Geometry: final body of the model. Coordinates: model frame, mm. Give positions to 0.01 mm unless a question says otherwise; leave off trailing zeros. Order: outer loops, then holes, each group sorted by start corner. A loop starts at its lowest first (then second) coordinate and runs counter-clockwise, first axis right, second up. Notation, with made-up numbers: (-7, 13.25) -> (22, 13.25) arc R8 ccw to (22, 23.25) -> close; hole circle Ø11 at (79.5, -3). An arc over 180 degrees is marked (long way). Answer in a Markdown table with one row per item. Add a question column.
Q1. Cut plane C-C on x = -42. Return the cut outline in (y, z), and give its area (3 significant figures).
Q2. Line query: line 1 along X through (y, z) = (3.7, 52); line 2 along X through (y, z) = (2.5, 130.5); line 3 along Z through (x, y) = (-10.5, 1.55). Output: solid intervals per line, ascending. Write a range as from..to.
Q3. Cut plane A-A on z = 45. Return the cut outline in (x, y).
Q4. Cut plane B-B on x = 21.5. Return the cut outline in (y, z), and give its area (3 significant figures).
Q5. Contact query for flat-ended pins moving along their axis: P1, Ø1.5, axis at y = 2, z = 129, coming from the +X side; P2, Ø3, axis at x = -34.5, y = 1.5, coming from the +Z side; P3, Ø2.5, axis at x = 0.5, y = 3.5, coming from the -Z side. Output: stop coordinate, or through.
Q6. Cut plane D-D on z = 73. Return the cut outline in (x, y).
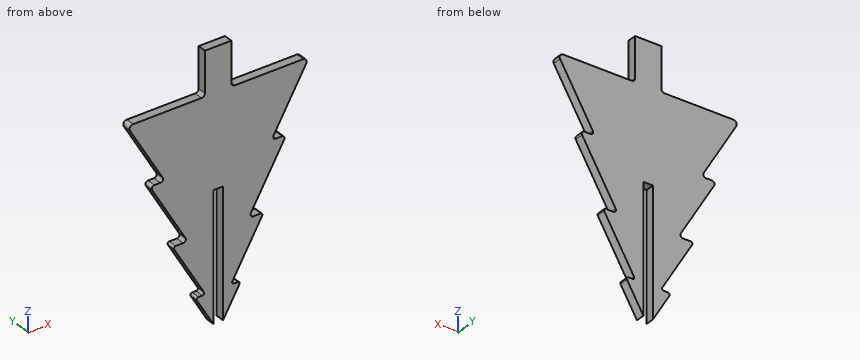
from build123d import *

# Parameters (mm, degrees)
ESBO_O1_W     = 15
ESBO_O1_H     = 25
RVORE_DEPTH   = 5
ESBO_O3_W     = 5.5
ESBO_O3_H     = 77.5
ENCAIXE_DEPTH = 5
FILETE1_R     = 1.5
FILETE2_R     = 1
FILETE3_R     = 1.5
FILETE4_R     = 1.5
FILETE5_R     = 2
FILETE6_R     = 1
FILETE7_R     = 1
FILETE8_R     = 2
FILETE9_R     = 1.5
FILETE10_R    = 1.5
FILETE11_R    = 1.5
FILETE12_R    = 1
FILETE13_R    = 1
FILETE14_R    = 1
FILETE15_R    = 2
FILETE16_R    = 2


with BuildPart() as part:
    # Esboço1 → rvore (new body)
    with BuildSketch(Plane(origin=(0, 0, 0), x_dir=(1, 0, 0), z_dir=(0, 1, 0))):
        with Locations((0, -127.5)):
            Rectangle(ESBO_O1_W, ESBO_O1_H)
        Polygon((-51.961524227, -115), (-7.5, -115), (7.5, -115), (51.961524227, -115), (30.310889132, -77.5), (-30.310889132, -77.5), align=None)
        Polygon((-8.660254038, -40), (-30.310889132, -77.5), (30.310889132, -77.5), (8.660254038, -40), align=None)
        Polygon((-17.320508076, -40), (-8.660254038, -40), (0, -25), (8.660254038, -40), (17.320508076, -40), (0, -10), align=None)
        Polygon((8.660254038, -40), (30.310889132, -77.5), (38.97114317, -77.5), (17.320508076, -40), align=None)
        Polygon((0, -25), (-8.660254038, -40), (8.660254038, -40), align=None)
        Polygon((-38.97114317, -77.5), (-30.310889132, -77.5), (-8.660254038, -40), (-17.320508076, -40), align=None)
        Polygon((-25.980762114, -40), (-17.320508076, -40), (0, -10), (17.320508076, -40), (25.980762114, -40), (7.216878365, -7.5), (-7.216878365, -7.5), align=None)
        Polygon((0, 5), (-7.216878365, -7.5), (7.216878365, -7.5), align=None)
        Polygon((-12.990381057, -7.5), (-7.216878365, -7.5), (0, 5), (7.216878365, -7.5), (12.990381057, -7.5), (0, 15), align=None)
    extrude(amount=RVORE_DEPTH)

    # Esboço3 → Encaixe (cut)
    with BuildSketch(Plane(origin=(0, 5, 0), x_dir=(1, 0, 0), z_dir=(0, 1, 0))):
        with Locations((0, -23.75)):
            Rectangle(ESBO_O3_W, ESBO_O3_H)
    extrude(amount=-ENCAIXE_DEPTH, mode=Mode.SUBTRACT)

    # Filete1
    filete1_edges = [part.edges().sort_by_distance(p)[0] for p in [
        (17.320508076, 2.5, 40),
    ]]
    fillet(filete1_edges, radius=FILETE1_R)

    # Filete2
    filete2_edges = [part.edges().sort_by_distance(p)[0] for p in [
        (25.980762114, 2.5, 40),
    ]]
    fillet(filete2_edges, radius=FILETE2_R)

    # Filete3
    filete3_edges = [part.edges().sort_by_distance(p)[0] for p in [
        (38.97114317, 2.5, 77.5),
    ]]
    fillet(filete3_edges, radius=FILETE3_R)

    # Filete4
    filete4_edges = [part.edges().sort_by_distance(p)[0] for p in [
        (30.310889132, 2.5, 77.5),
    ]]
    fillet(filete4_edges, radius=FILETE4_R)

    # Filete5
    filete5_edges = [part.edges().sort_by_distance(p)[0] for p in [
        (51.961524227, 2.5, 115),
    ]]
    fillet(filete5_edges, radius=FILETE5_R)

    # Filete6
    filete6_edges = [part.edges().sort_by_distance(p)[0] for p in [
        (12.990381057, 2.5, 7.5),
    ]]
    fillet(filete6_edges, radius=FILETE6_R)

    # Filete7
    filete7_edges = [part.edges().sort_by_distance(p)[0] for p in [
        (7.216878365, 2.5, 7.5),
    ]]
    fillet(filete7_edges, radius=FILETE7_R)

    # Filete8
    filete8_edges = [part.edges().sort_by_distance(p)[0] for p in [
        (-51.961524227, 2.5, 115),
    ]]
    fillet(filete8_edges, radius=FILETE8_R)

    # Filete9
    filete9_edges = [part.edges().sort_by_distance(p)[0] for p in [
        (-30.310889132, 2.5, 77.5),
    ]]
    fillet(filete9_edges, radius=FILETE9_R)

    # Filete10
    filete10_edges = [part.edges().sort_by_distance(p)[0] for p in [
        (-38.97114317, 2.5, 77.5),
    ]]
    fillet(filete10_edges, radius=FILETE10_R)

    # Filete11
    filete11_edges = [part.edges().sort_by_distance(p)[0] for p in [
        (-17.320508076, 2.5, 40),
    ]]
    fillet(filete11_edges, radius=FILETE11_R)

    # Filete12
    filete12_edges = [part.edges().sort_by_distance(p)[0] for p in [
        (-25.980762114, 2.5, 40),
    ]]
    fillet(filete12_edges, radius=FILETE12_R)

    # Filete13
    filete13_edges = [part.edges().sort_by_distance(p)[0] for p in [
        (-7.216878365, 2.5, 7.5),
    ]]
    fillet(filete13_edges, radius=FILETE13_R)

    # Filete14
    filete14_edges = [part.edges().sort_by_distance(p)[0] for p in [
        (-12.990381057, 2.5, 7.5),
    ]]
    fillet(filete14_edges, radius=FILETE14_R)

    # Filete15
    filete15_edges = [part.edges().sort_by_distance(p)[0] for p in [
        (-7.5, 2.5, 115),
    ]]
    fillet(filete15_edges, radius=FILETE15_R)

    # Filete16
    filete16_edges = [part.edges().sort_by_distance(p)[0] for p in [
        (7.5, 2.5, 115),
    ]]
    fillet(filete16_edges, radius=FILETE16_R)


solid = part.part
Completed:
| question | item | result |
|---|---|---|
| 1 | outline | (0, 97.75) -> (5, 97.75) -> (5, 115) -> (0, 115) -> close |
| 1 | area | 86.3 mm² |
| 2 | line 1 | x = -24.25..-2.75, 2.75..24.25 |
| 2 | line 2 | x = -7.5..7.5 |
| 2 | line 3 | z = 3.19..7.5, 13.19..115 |
| 3 | outline | (-20.21, 0) -> (-2.75, 0) -> (-2.75, 5) -> (-20.21, 5) -> close; (2.75, 0) -> (20.21, 0) -> (20.21, 5) -> (2.75, 5) -> close |
| 4 | outline | (0, 32.24) -> (5, 32.24) -> (5, 40) -> (0, 40) -> close; (0, 47.24) -> (5, 47.24) -> (5, 115) -> (0, 115) -> close |
| 4 | area | 378 mm² |
| 5 | P1 | stops at x = 7.5 |
| 5 | P2 | stops at z = 115 |
| 5 | P3 | stops at z = 62.5 |
| 6 | outline | (-36.37, 0) -> (36.37, 0) -> (36.37, 5) -> (-36.37, 5) -> close |
